```python
from build123d import *

# Parameters (mm, degrees)
EXTRUDE_1_DEPTH     = 2000
EXTRUDE_2_DEPTH     = 1900
EXTRUDE_START       = -10
EXTRUDE_3_DEPTH     = 10
SKETCH_4_R          = 4
CUT_EXTRUDE_1_DEPTH = 10


with BuildPart() as part:
    # 草图1 → 凸台-拉伸1 (new body)
    with BuildSketch(Plane(origin=(0, 0, 0), x_dir=(1, 0, 0), z_dir=(0, 1, 0))):
        with BuildLine():
            Line((0, 1540), (0, 1515))
            ThreePointArc((0, 1515), (210.847247954, 1500.256124143), (417.590594063, 1456.311469347))
            Line((417.590594063, 1456.311469347), (424.481527958, 1480.343011745))
            ThreePointArc((424.481527958, 1480.343011745), (214.326575478, 1525.012825862), (0, 1540))
        make_face()
    extrude(amount=EXTRUDE_1_DEPTH)

    # 草图2 → 凸台-拉伸2 (add)
    with BuildSketch(Plane(origin=(0, 2000, 0), x_dir=(1, 0, 0), z_dir=(0, 1, 0))):
        Polygon((475.59627434, 1463.734823878), (424.481527958, 1480.343011745), (417.590594063, 1456.311469347), (454.15659952, 1444.430453961), align=None)
    extrude(amount=-EXTRUDE_2_DEPTH)

    # 草图3 → 凸台-拉伸3 (add)
    with BuildSketch(Plane(origin=(0, 1970.4, 0), x_dir=(1, 0, 0), z_dir=(0, 1, 0)).offset(EXTRUDE_START)):
        with BuildLine():
            Line((201.678827868, 1501.516117259), (194.962988272, 1451.516117259))
            ThreePointArc((194.962988272, 1451.516117259), (232.892441695, 1445.915182873), (270.662282272, 1439.323290444))
            Line((270.662282272, 1439.323290444), (279.985715854, 1488.903287295))
            ThreePointArc((279.985715854, 1488.903287295), (240.914827355, 1495.722248935), (201.678827868, 1501.516117259))
        make_face()
    extrude(amount=EXTRUDE_3_DEPTH)

    # 草图4 → 切除-拉伸1 (cut)
    with BuildSketch(Plane(origin=(0, 1970.4, 0), x_dir=(1, 0, 0), z_dir=(0, 1, 0))):
        with Locations(Location((217.889718701, 1464.147071856, 0), (0, 0, 270))):
            Circle(SKETCH_4_R)
    extrude(amount=-CUT_EXTRUDE_1_DEPTH, mode=Mode.SUBTRACT)


solid = part.part
```
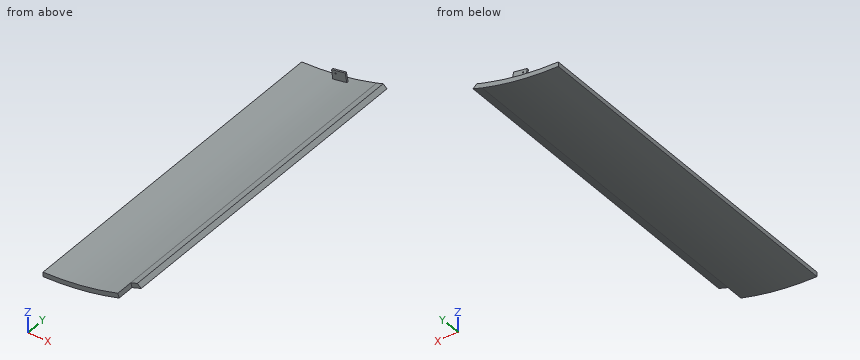
Design review of the part built by this model. Coordinates are the model's own, in mm. Give positions to 0.01 mm unless a question says otherwise; leave off trailing zeros. Order: outer loops, then holes, each group sorted by start corner. A loop starts at its lowest first (then second) coordinate and runs counter-clockwise, first axis right, second up. Notation, with made-up numbers: M -39.5,-2.75 L -9.5,-2.75 A8 cw -9.5,9.25 Z; hole C -12,10.5 d2. An arc over 180 degrees is marked long. One line per question, with ' | ' between items. Start each with the question number.
Q1. We need section C-C (x = 321). Write out the cut boundary in (y, z).
Q2. For pin 1 Ø5 at (x, y) = (207.5, 1632) entering from +Z; pin 2 Ø11 at (x, z) = (436.5, -1467.5) entering from -Y; pin 3 Ø9 at (x, z) = (217.89, -1464.15) entering from +Y, all flat-tipped, find the tip position at first contact; note any pin that passes through.
Q3. We need section D-D (x = 399). Write out the cut boundary in (y, z).
Q4. We need section B-B (x = 241). Write out the cut boundary in (y, z), plus the area to 3 significant figures.
Q5. We need section A-A (y = 1073). Write out the cut boundary in (x, z).
Q6. For L1, parallel to Y at x = 227.5, z = -1496.5; L2, parallel to Z at x = 20, y = 731; L3, parallel to Z at x = 164, y = 1496.5, list the stretches that pass through material, from the lowest coordinate up. Write a range as [from, to].
Returned:
1) outline: M 0,-1506.17 L 2000,-1506.17 L 2000,-1480.6 L 0,-1480.6 Z
2) pin 1: z = -1500.37 | pin 2: y = 100 | pin 3: y = 1970.4
3) outline: M 0,-1487.41 L 2000,-1487.41 L 2000,-1461.51 L 0,-1461.51 Z
4) outline: M 0,-1521.03 L 2000,-1521.03 L 2000,-1495.71 L 1970.4,-1495.71 L 1970.4,-1444.59 L 1960.4,-1444.59 L 1960.4,-1495.71 L 0,-1495.71 Z | area: 51,100 mm2
5) outline: M 0,-1540 A1540 ccw 424.48,-1480.34 L 475.6,-1463.73 L 454.16,-1444.43 L 417.59,-1456.31 A1515 cw 0,-1515 Z
6) L1: [1960.4, 1970.4] | L2: [-1539.87, -1514.87] | L3: [-1531.24, -1506.1]
